Geometry check sheet. Reference: the model listing, model coordinates, mm. Face numbers are marked on the shaded views. A direction names the side the tool comes from. Round coordinates to 2 decimals unless told otherwise and drop trailing zeros. Write each loop counter-clockwise with the first axis right and the second up, starting at its lowest first coordinate (ties: lowest second). Pieces come first, ordered by that corner, then holes.
Item 1: Cross-section at B-B (y = 15). Enter the section's corners in (x, z).
Item 2: Cross-section at D-D (x = 30.5). Enter the section's corners in (y, z), then the cut area to 3 significant figures.
Item 3: Cross-section at A-A (x = 3). Enter the section's corners in (y, z), then the cut area to 3 significant figures.
Item 4: Scan lines: probe 1 along X at (y, z) = (14, 24); probe 2 along Z at (x, y) = (1, 15). Record each from-to range of solid material in increasing order.
Item 5: Depth check by flat-ended pin: P1, Ø8, axis at y = 16, z = 14, coming from the +X side; P2, Ø5, axis at x = 30.5, y = 12.5, coming from the +Z side; P3, Ø8.5, axis at x = 15.5, z = 15.5, coming from the +Y side. Enter the tip coordinate at first touch or a pass-through.
Item 6: Cross-section at C-C (z = 15). Enter the section's corners in (x, y).
Item 7: Draft check along X on the marked faces 1, 2 and 3. Enter one of: pulls with the +X half, pulls with the -X half, needs draft (parallel to the pull), parting line crosses it, or undercut.
Item 8: Access from +Z, -Z, +X, -X, +Y, -Y to the whole of each face (thin tool, end or side, straight path). Record for the marked faces 4, 5 and 6.
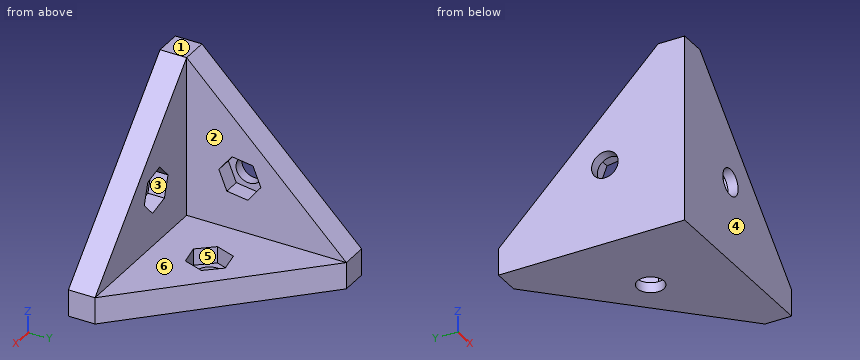
from build123d import *

# Parameters (mm, degrees)
SKETCH_R        = 2.5
PAD_DEPTH       = 5
SKETCH001_R     = 2.5
PAD001_DEPTH    = 5
SKETCH002_R     = 2.5
PAD002_DEPTH    = 5
POCKET_DEPTH    = 3.1
POCKET001_DEPTH = 3.1
POCKET002_DEPTH = 3.1


with BuildPart() as part:
    # Sketch → Pad (new body)
    with BuildSketch(Plane.XY):
        Polygon((0, 0), (0, 35), (5, 35), (35, 5), (35, 0), align=None)
        with Locations((15, 15)):
            Circle(SKETCH_R, mode=Mode.SUBTRACT)
    extrude(amount=PAD_DEPTH)

    # Sketch001 → Pad001 (join)
    with BuildSketch(Plane.XZ):
        Polygon((0, 0), (0, 35), (5, 35), (35, 5), (35, 0), align=None)
        with Locations((15, 15)):
            Circle(SKETCH001_R, mode=Mode.SUBTRACT)
    extrude(amount=-PAD001_DEPTH)

    # Sketch002 → Pad002 (join)
    with BuildSketch(Plane.YZ):
        Polygon((0, 0), (0, 35), (5, 35), (35, 5), (35, 0), align=None)
        with Locations((15, 15)):
            Circle(SKETCH002_R, mode=Mode.SUBTRACT)
    extrude(amount=PAD002_DEPTH)

    # Sketch003 (on Face11 of Pad002) → Pocket (cut)
    with BuildSketch(Plane(origin=(0, 5, 0), x_dir=(-1, 0, 0), z_dir=(0, 1, 0))):
        Polygon((-13.828396, 18.807538), (-17.711622, 17.918408), (-18.883227, 14.11087), (-16.171604, 11.192462), (-12.288378, 12.081592), (-11.116773, 15.88913), align=None)
    extrude(amount=-POCKET_DEPTH, mode=Mode.SUBTRACT)

    # Sketch004 (on Face10 of Pocket) → Pocket001 (cut)
    with BuildSketch(Plane.XY.offset(5)):
        Polygon((16.321291, 18.758216), (12.405934, 18.023379), (11.084644, 14.265163), (13.678709, 11.241784), (17.594066, 11.976621), (18.915356, 15.734837), align=None)
    extrude(amount=-POCKET001_DEPTH, mode=Mode.SUBTRACT)

    # Sketch005 (on Face12 of Pocket001) → Pocket002 (cut)
    with BuildSketch(Plane.YZ.offset(5)):
        Polygon((18.944452, 14.442056), (17.45542, 18.137023), (13.510968, 18.694967), (11.055548, 15.557944), (12.54458, 11.862977), (16.489032, 11.305033), align=None)
    extrude(amount=-POCKET002_DEPTH, mode=Mode.SUBTRACT)


solid = part.part
Resolved:
1. outline: (0, 0) - (12.5, 0) - (12.5, 1.9) - (11.34, 1.9) - (11.34, 5) - (5, 5) - (5, 11.52) - (1.9, 11.52) - (1.9, 12.5) - (0, 12.5) - close; (0, 17.5) - (1.9, 17.5) - (1.9, 18.48) - (5, 18.48) - (5, 25) - (0, 25) - close; (17.5, 0) - (25, 0) - (25, 5) - (18.66, 5) - (18.66, 1.9) - (17.5, 1.9) - close
2. outline: (0, 0) - (9.5, 0) - (9.5, 5) - (5, 5) - (5, 9.5) - (0, 9.5) - close
2. area: 70.0 mm2
3. outline: (0, 0) - (35, 0) - (35, 5) - (5, 35) - (0, 35) - close; hole (11.06, 15.56) - (12.54, 11.86) - (16.49, 11.31) - (18.94, 14.44) - (17.46, 18.14) - (13.51, 18.69) - close
3. area: 734 mm2
4. probe 1: x = 0 to 5
4. probe 2: z = 0 to 12.5, 17.5 to 25
5. P1: stops at x = 5
5. P2: stops at z = 5
5. P3: stops at y = 5
6. outline: (0, 0) - (12.5, 0) - (12.5, 1.9) - (11.39, 1.9) - (11.39, 5) - (5, 5) - (5, 11.28) - (1.9, 11.28) - (1.9, 12.5) - (0, 12.5) - close; (0, 17.5) - (1.9, 17.5) - (1.9, 18.72) - (5, 18.72) - (5, 25) - (0, 25) - close; (17.5, 0) - (25, 0) - (25, 5) - (18.61, 5) - (18.61, 1.9) - (17.5, 1.9) - close
7. face 1: needs draft
7. face 2: pulls with the +X half
7. face 3: undercut
8. face 4: +Z, -Z, +X, -X, -Y
8. face 5: +Z
8. face 6: +Z, +X, +Y
